Build history of the part. All positions in model axes, mm. A direction names the side the tool comes from. Round coordinates to 2 decimals unless told otherwise and drop trailing zeros. Loops run counter-clockwise (first coordinate to the right, second up) from the corner with the lowest first, then second, coordinate; pieces in that order, holes last. Notation, with made-up numbers: (71, 57.5) - (93, 57.5) arc R21 ccw to (93, 96.5) - close; hole circle Ø10 at (2.5, 23.5). An arc over 180 degrees is marked (long way). One line per question, with ' | ' between items. Start each with the question number.
Autodesk Inventor part; units mm, degrees
ref_plane "YZ Plane" through (0, 0, 0) normal (1, 0, 0) x (0, 1, 0)
ref_plane "XZ Plane" through (0, 0, 0) normal (0, 1, 0) x (-1, 0, 0)
ref_plane "XY Plane" through (0, 0, 0) normal (0, 0, 1) x (1, 0, 0)
sketch "Sketch1" plane through (0, 0, 0) normal (0, 0, 1) x (1, 0, 0)
  line L0 (91.3955, 137.1362) -> (100.6455, 137.1362) construction
  line L1 (100.6455, 137.1362) -> (100.6455, 129.3358)
  line L2 (100.6455, 137.1362) -> (100.6455, 144.9367)
  line L3 (91.3955, 137.1362) -> (91.3955, 122.6202) construction
  line L4 (82.1455, 137.1362) -> (82.1455, 129.3358)
  line L5 (82.1455, 137.1362) -> (82.1455, 144.9367)
  arc A0 (100.6455, 144.9367) -> (82.1455, 144.9367) centre (91.3955, 137.1362) ccw
  arc A1 (82.1455, 129.3358) -> (100.6455, 129.3358) centre (91.3955, 137.1362) ccw
  point P0 (0, 0)
  point P1 (100.6455, 120.0736)
  point P2 (100.6455, 151.3606)
  point P3 (82.1455, 120.0736)
  point P4 (82.1455, 151.3606)
  dimension "d1" = 9.25
extrude "Extrusion1" add sketch "Sketch1" along normal blind 36
sketch "Sketch2" plane through (0, 0, 36) normal (0, 0, 1) x (1, 0, 0)
  arc A0 (100.6455, 144.9367) -> (82.1455, 144.9367) centre (91.3955, 137.1362) ccw
  circle A1 centre (91.3955, 137.1362) radius 2.3
  point P0 (0, 0)
  dimension "d4" = 4.6
extrude "Extrusion2" add sketch "Sketch2" along normal blind 13
properties part number "motor_12v"
1) Tool access for faces 1 (the flat face through (100.646, 137, 18)), 2 (the cylindrical face through (90.897, 139.382, 42.409)): list every direction of +Z, -Z, +X, -X, +Y, -Y with a clear straight run to the whole face (end or side of a thin tool).
2) Saw through at C-C on y = 143. Write the cut outline in (x, z), and give its area (3 significant figures).
3) Saw through at D-D on z = 38.5. Write the cut outline in (x, y).
4) Drop flat-ended pins along their axis: pin 1 (1 mm diameter, centred on x = 84.5, y = 137.5, fed in from +Z); pin 2 (6 mm diameter, centred on x = 97.5, z = 32.5, fed in from +Y). Give the stop position or say it passes through.
5) Saw through at A-A on x = 90. Write the cut outline in (y, z).
6) Saw through at B-B on z = 25.5. Write the cut outline in (x, y).
7) Wall check: line 1 (Z direction, x = 87.75, y = 132.5); line 2 (Y direction, x = 91.25, z = 21.5); line 3 (X direction, y = 126.25, z = 17). Give the ranges that are in metal, low to high. Write a range as [from, to].
Answer key:
1) face 1: +Z, -Z, +X, +Y, -Y | face 2: +Z
2) outline: (82.15, 0) - (100.65, 0) - (100.65, 36) - (82.15, 36) - close | area: 666 mm²
3) outline: circle Ø4.6 at (91.4, 137.14)
4) pin 1: z = 36 | pin 2: y = 148.83
5) outline: (125.12, 0) - (149.16, 0) - (149.16, 36) - (138.96, 36) - (138.96, 49) - (135.31, 49) - (135.31, 36) - (125.12, 36) - close
6) outline: (82.15, 129.34) arc R12.1 ccw to (100.65, 129.34) - (100.65, 144.94) arc R12.1 ccw to (82.15, 144.94) - close
7) line 1: [0, 36] | line 2: [125.04, 149.24] | line 3: [86.11, 96.68]
